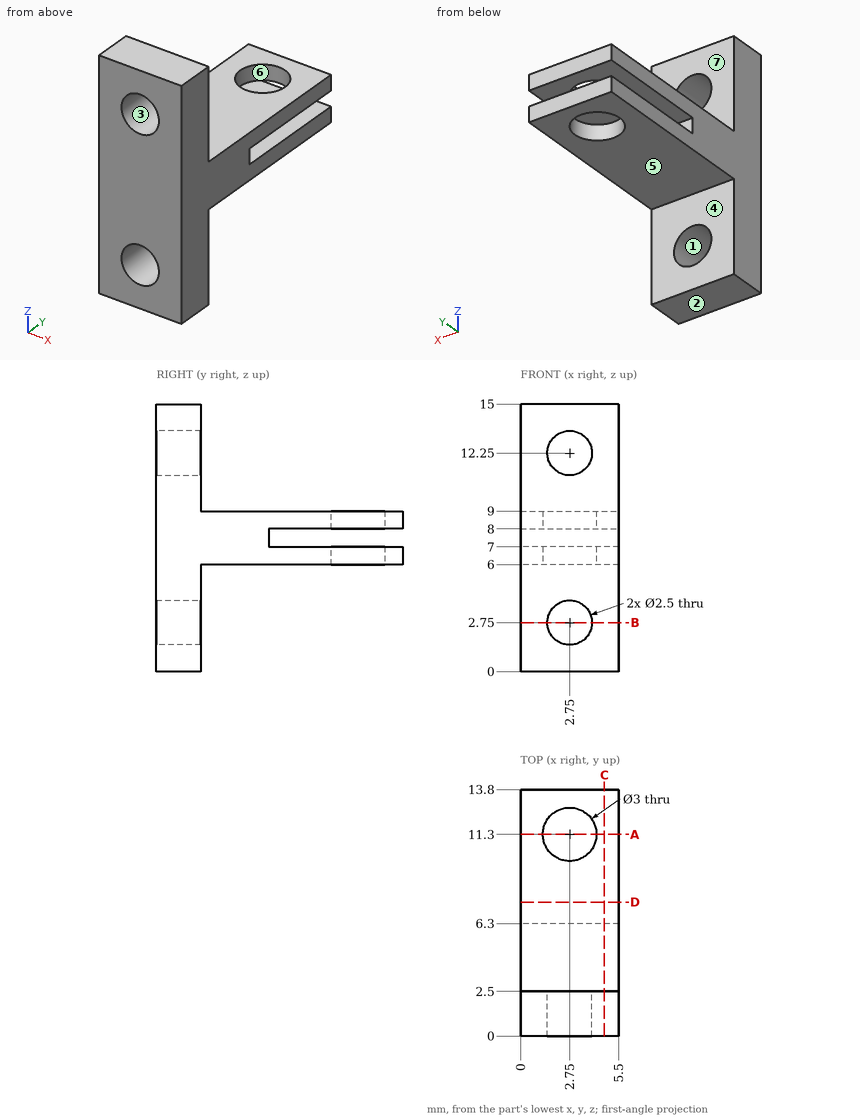
Study the drawing (mm; zero at the part's minimum x, y, z) and answer. A direction names the side the tool comes from. Give positions to 0.01 mm unless a question says otherwise; leave off trailing zeros. Loops run counter-clockwise (first coordinate to the right, second up) from the corner with the lowest first, then second, coordinate; pieces in that order, holes last. Notation, with made-up numbers: (-6.5, 24) - (26.5, 24) arc R13 ccw to (26.5, 29) - close; hole circle Ø2 at (88, -12). An arc over 180 degrees is marked (long way). Answer as CSV lines item,"result". Start each with the question number.
1) Straight lines are drawn through the part: L1, parallel to X at y = 2, z = 12.25; L2, parallel to Z at x = 1.45, y = 3.25; L3, parallel to Y at x = 1.45, z = 7.25. For each, find the intervals that lie inside material, in ascending order. Write a range as from..to.
2) Find section C-C (x = 4.7). Write down the section's boundary in (y, z).
3) Determine the mould class of the marked faces 1, 2, 3 and 4 for opening direction Z: released by +Z, released by -Z, zero draft, split by the parting line, or undercut.
4) Each of these flat-tipped pins is pushed along its axis until it touches: pin 1 Ø3 at (x, y) = (3, 5.5) entering from +Z; pin 2 Ø2 at (x, y) = (1.5, 12) entering from -Z; pin 3 Ø0.5 at (x, z) = (2, 7.5) entering from +Y. Where does it stop, or does it pass through?
5) Find section B-B (z = 2.75). Write down the section's boundary in (x, y), then the cut area to 3 significant figures.
6) Find section D-D (y = 7.5). Write down the section's boundary in (x, z), then the cut area to 3 significant figures.
7) Which of the six approach directions +Z, -Z, +X, -X, +Y, -Y give full straight-line access (tool end or side, diameter ignored) to the marked faces 5, 6 and 7?
8) Find section A-A (y = 11.3). Write down the section's boundary in (x, z).
Findings below:
1,L1,"0..1.5, 4..5.5"
1,L2,"6..9"
1,L3,"0..6.3"
2,outline,"(0, 0) - (2.5, 0) - (2.5, 6) - (13.8, 6) - (13.8, 7) - (6.3, 7) - (6.3, 8) - (13.8, 8) - (13.8, 9) - (2.5, 9) - (2.5, 15) - (0, 15) - close"
3,face 1,"undercut"
3,face 2,"released by -Z"
3,face 3,"undercut"
3,face 4,"zero draft"
4,pin 1,"z = 9"
4,pin 2,"z = 6"
4,pin 3,"y = 6.3"
5,outline,"(0, 0) - (1.5, 0) - (1.5, 2.5) - (0, 2.5) - close; (4, 0) - (5.5, 0) - (5.5, 2.5) - (4, 2.5) - close"
5,area,"7.50 mm^2"
6,outline,"(0, 6) - (5.5, 6) - (5.5, 7) - (0, 7) - close; (0, 8) - (5.5, 8) - (5.5, 9) - (0, 9) - close"
6,area,"11.0 mm^2"
7,face 5,"-Z, +X, -X, +Y"
7,face 6,"+Z, -Z"
7,face 7,"+Z, +X, -X, +Y"
8,outline,"(0, 6) - (1.25, 6) - (1.25, 7) - (0, 7) - close; (0, 8) - (1.25, 8) - (1.25, 9) - (0, 9) - close; (4.25, 6) - (5.5, 6) - (5.5, 7) - (4.25, 7) - close; (4.25, 8) - (5.5, 8) - (5.5, 9) - (4.25, 9) - close"
